Work out the finished part from the listing and answer in its coordinate system (mm). Face numbers are marked on the shaded views. Round coordinates to 2 decimals unless told otherwise and drop trailing zeros. Loops run counter-clockwise (first coordinate to the right, second up) from the corner with the lowest first, then second, coordinate; pieces in that order, holes last.
```python
from build123d import *

# Parameters (mm, degrees)
SKETCH1_W            = 10
SKETCH1_H            = 30
SKETCH1_W_2          = 30
BOSS_EXTRUDE4_DEPTH  = 7
SKETCH3_W            = 30
SKETCH3_H            = 30
BOSS_EXTRUDE5_DEPTH  = 3
SKETCH4_W            = 7
SKETCH4_H            = 7
BOSS_EXTRUDE8_DEPTH  = 50
SKETCH6_R            = 2
BOSS_EXTRUDE9_DEPTH  = 20
SKETCH7_W            = 7
SKETCH7_H            = 7
BOSS_EXTRUDE13_DEPTH = 100
SKETCH10_R           = 2
BOSS_EXTRUDE14_DEPTH = 20


with BuildPart() as part:
    # Sketch1 → Boss-Extrude4 (new body)
    with BuildSketch(Plane.XY):
        with Locations((-20, 0)):
            Rectangle(SKETCH1_W, SKETCH1_H)
        Rectangle(SKETCH1_W_2, SKETCH1_H)
        with Locations((20, 0)):
            Rectangle(SKETCH1_W, SKETCH1_H)
    extrude(amount=BOSS_EXTRUDE4_DEPTH)

    # Sketch3 → Boss-Extrude5 (add)
    with BuildSketch(Plane(origin=(0, 0, 0), x_dir=(-1, 0, 0), z_dir=(0, 0, -1))):
        Rectangle(SKETCH3_W, SKETCH3_H)
    extrude(amount=BOSS_EXTRUDE5_DEPTH)

    # Sketch4 → Boss-Extrude8 (add)
    with BuildSketch(Plane(origin=(0, 0, -3), x_dir=(-1, 0, 0), z_dir=(0, 0, -1))):
        with Locations((-6.620919375, -4.848854148)):
            Rectangle(SKETCH4_W, SKETCH4_H)
    extrude(amount=BOSS_EXTRUDE8_DEPTH)

    # Sketch6 → Boss-Extrude9 (add)
    with BuildSketch(Plane(origin=(0, -1.348854148, 0), x_dir=(1, 0, 0), z_dir=(0, 1, 0))):
        with Locations((6.620919375, 45.83776359)):
            Circle(SKETCH6_R)
    extrude(amount=BOSS_EXTRUDE9_DEPTH)

    # Sketch7 → Boss-Extrude13 (add)
    with BuildSketch(Plane(origin=(0, 0, -3), x_dir=(-1, 0, 0), z_dir=(0, 0, -1))):
        with Locations((7.796290003, -4.848854148)):
            Rectangle(SKETCH7_W, SKETCH7_H)
    extrude(amount=BOSS_EXTRUDE13_DEPTH)

    # Sketch10 → Boss-Extrude14 (add)
    with BuildSketch(Plane(origin=(0, -1.348854148, 0), x_dir=(1, 0, 0), z_dir=(0, 1, 0))):
        with Locations((-7.583363056, 97.696042798)):
            Circle(SKETCH10_R)
    extrude(amount=BOSS_EXTRUDE14_DEPTH)


solid = part.part
```
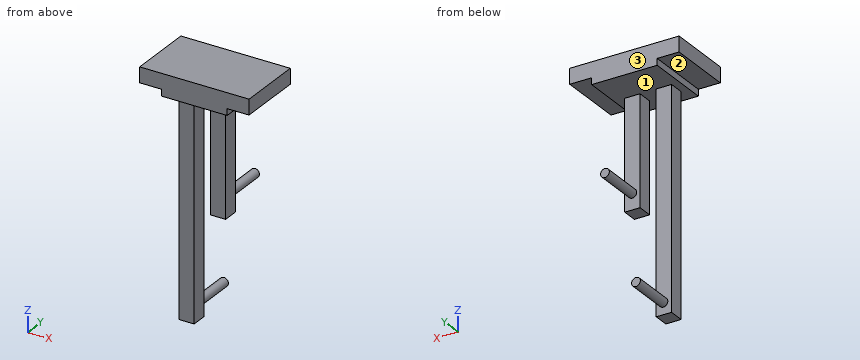
1. Determine the mould class of the marked faces 1, 2 and 3 for opening direction Z: +Z half, -Z half, draft (parallel to the pull), parting line (faces both ways), or undercut.
Answer key:
face 1: undercut
face 2: -Z half
face 3: draft
2. Consider probe 1 along X at (y, z) = (-3, -14); probe 2 along Z at (x, y) = (-9, -11); probe 3 along Y at (x, z) = (-11, -23). Determine where each line is inside the solid, lowest interval first.
Answer key:
probe 1: x = -11.3 to -4.3, 3.12 to 10.12
probe 2: z = -3 to 7
probe 3: y = -8.35 to -1.35
3. Find section C-C (x = 6). Write down the section's boundary in (y, z).
Answer key:
outline: (-15, -3) - (-8.35, -3) - (-8.35, -53) - (-1.35, -53) - (-1.35, -47.74) - (18.65, -47.74) - (18.65, -43.94) - (-1.35, -43.94) - (-1.35, -3) - (15, -3) - (15, 7) - (-15, 7) - close
4. Given pin 1 (6 mm diameter, centred on y = -9.5, z = -57, fed in from -X); pin 2 (3 mm diameter, centred on x = -19, y = 4.5, fed in from -Z); pin 3 (5.5 mm diameter, centred on x = -8, z = -73.5, fed in from -Y), each flat-ended and moving along its own axis, determine where each tip first touches the part or whether it passes through.
Answer key:
pin 1: stops at x = -11.3
pin 2: stops at z = 0
pin 3: stops at y = -8.35
5. Find section A-A (z = -34). Write down the section's boundary in (x, y).
Answer key:
outline: (-11.3, -8.35) - (-4.3, -8.35) - (-4.3, -1.35) - (-11.3, -1.35) - close; (3.12, -8.35) - (10.12, -8.35) - (10.12, -1.35) - (3.12, -1.35) - close
6. Find section D-D (y = 7.5). Write down the section's boundary in (x, z), then the cut area to 3 significant figures.
Answer key:
outline: (-25, 0) - (-15, 0) - (-15, -3) - (15, -3) - (15, 0) - (25, 0) - (25, 7) - (-25, 7) - close; circle Ø4 at (-7.58, -97.7); circle Ø4 at (6.62, -45.84)
area: 465 mm2
7. Find section B-B (y = -5). Write down the section's boundary in (x, z).
Answer key:
outline: (-25, 0) - (-15, 0) - (-15, -3) - (-11.3, -3) - (-11.3, -103) - (-4.3, -103) - (-4.3, -3) - (3.12, -3) - (3.12, -53) - (10.12, -53) - (10.12, -3) - (15, -3) - (15, 0) - (25, 0) - (25, 7) - (-25, 7) - close
